Study the drawing (mm; zero at the part's minimum x, y, z) and answer. Coordinates: 2 decimals unless noted, no trailing zeros. Order: outer loops, then holes, each group sorted by start corner. A loop starts at its lowest first (then second) coordinate and runs counter-clockwise, first axis right, second up. Notation, with made-up numbers: (37, -30.5) -> (62, -30.5) arc R14 ccw to (62, -22.5) -> close; hole circle Ø6 at (73, 46). An arc over 180 degrees is marked (long way). Answer as CSV lines item,"result". Start each with the question number.
Item 1: Section C-C (y = 17) is taken. Write down the section's boundary in (x, z).
Item 2: Straight lines are drawn through the part: L1, parallel to X at y = 8.5, z = 1.9; L2, parallel to X at y = 18, z = 1.6; L3, parallel to X at y = 23.5, z = 0.5. For each, find the intervals that lie inside material, in ascending order.
Item 3: Section A-A (x = 37) is taken. Write down the section's boundary in (y, z).
Item 4: Each of these flat-tipped pins is pushed along its axis until it touches: pin 1 Ø1 at (x, z) = (1, 0.5) entering from -Y; pin 2 Ø1 at (y, z) = (22, 1.5) entering from +X. Where does it stop, or does it pass through?
Item 5: Section B-B (z = 1.05) is taken. Write down the section's boundary in (x, y), then the cut area to 3 significant figures.
Item 6: Section D-D (y = 7) is taken. Write down the section's boundary in (x, z).
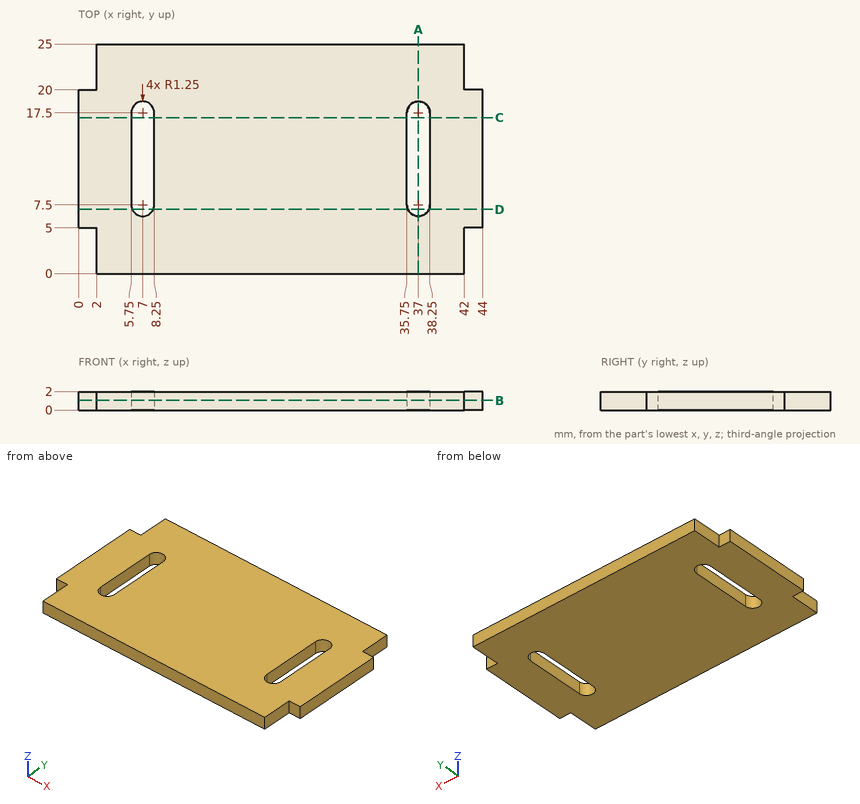
Checked values:
1,outline,"(0, 0) -> (5.75, 0) -> (5.75, 2) -> (0, 2) -> close; (8.25, 0) -> (35.75, 0) -> (35.75, 2) -> (8.25, 2) -> close; (38.25, 0) -> (44, 0) -> (44, 2) -> (38.25, 2) -> close"
2,L1,"x = 0 to 5.75, 8.25 to 35.75, 38.25 to 44"
2,L2,"x = 0 to 5.85, 8.15 to 35.85, 38.15 to 44"
2,L3,"x = 2 to 42"
3,outline,"(0, 0) -> (6.25, 0) -> (6.25, 2) -> (0, 2) -> close; (18.75, 0) -> (25, 0) -> (25, 2) -> (18.75, 2) -> close"
4,pin 1,"stops at y = 5"
4,pin 2,"stops at x = 42"
5,outline,"(0, 5) -> (2, 5) -> (2, 0) -> (42, 0) -> (42, 5) -> (44, 5) -> (44, 20) -> (42, 20) -> (42, 25) -> (2, 25) -> (2, 20) -> (0, 20) -> close; hole (5.75, 7.5) arc R1.25 ccw to (8.25, 7.5) -> (8.25, 17.5) arc R1.25 ccw to (5.75, 17.5) -> close; hole (35.75, 7.5) arc R1.25 ccw to (38.25, 7.5) -> (38.25, 17.5) arc R1.25 ccw to (35.75, 17.5) -> close"
5,area,"1,000 mm^2"
6,outline,"(0, 0) -> (5.85, 0) -> (5.85, 2) -> (0, 2) -> close; (8.15, 0) -> (35.85, 0) -> (35.85, 2) -> (8.15, 2) -> close; (38.15, 0) -> (44, 0) -> (44, 2) -> (38.15, 2) -> close"
